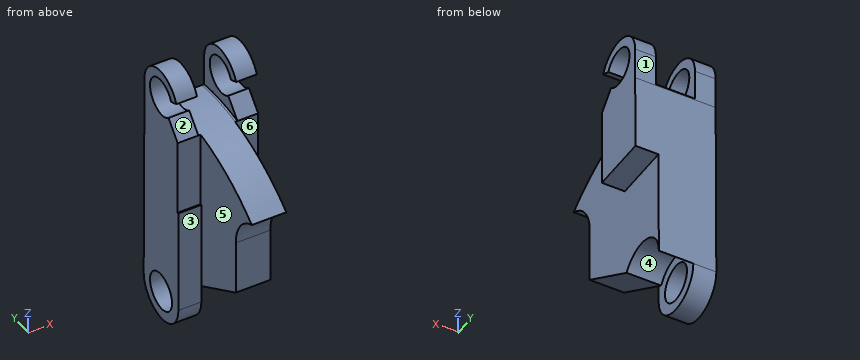
Autodesk Inventor part; units mm, degrees
ref_plane "YZ Plane" through (0, 0, 0) normal (1, 0, 0) x (0, 1, 0)
ref_plane "XZ Plane" through (0, 0, 0) normal (0, 1, 0) x (-1, 0, 0)
ref_plane "XY Plane" through (0, 0, 0) normal (0, 0, 1) x (1, 0, 0)
sketch "スケッチ1" plane through (0, 0, 0) normal (1, 0, 0) x (0, 1, 0)
  line L0 (0, 0) -> (0, 6)
  line L1 (0, 6) -> (0, -6)
  line L2 (0, 0) -> (11.5, 0)
  line L3 (11.5, 0) -> (11.5, 9.5)
  line L4 (11.5, 9.5) -> (11.5, -9.5)
  circle A0 centre (0, 6) radius 1.25
  circle A1 centre (0, -6) radius 1.25
  circle A2 centre (11.5, 9.5) radius 1.65
  circle A3 centre (11.5, -9.5) radius 1.65
  circle A4 centre (11.5, 9.5) radius 2.5
  circle A5 centre (11.5, -9.5) radius 2.5
  circle A6 centre (0, 0) radius 2.65
  line L5 (0, 0) -> (-14.6, 0)
  circle A7 centre (-14.6, 0) radius 1.65
  circle A8 centre (-14.6, 0) radius 2.5
  circle A9 centre (0, 6) radius 2
  circle A10 centre (0, -6) radius 2
  line L6 (0, 8) -> (10.6499, 11.851)
  line L7 (0, -8) -> (10.6499, -11.851)
  line L8 (-14.6, 0) -> (-14.6, -2.5)
  line L9 (-14.6, 0) -> (-12.1, 0) construction
  line L10 (-14.6, -2.5) -> (-14.6, 2.5)
  line L11 (-14.6, -2.5) -> (-0.7212, -7.8655)
  line L12 (-14.6, 2.5) -> (-0.7212, 7.8655)
  circle A11 centre (11.5, -9.5) radius 14.9164
  line L13 (11.5, -9.5) -> (0, 0)
  line L14 (11.5, -9.5) -> (0, -2.65)
  line L15 (14, 9.5) -> (14, 6.6979)
  circle A12 centre (11.5, -9.5) radius 16.7294
  circle A13 centre (11.5, -9.5) radius 2.6
  circle A14 centre (11.5, -9.5) radius 16.5
  line L16 (14, 6.6979) -> (14.1, -9.4839)
  line L17 (8.9, -9.5) -> (8.9, 0)
  line L18 (9, 9.5) -> (9, 0)
  line L19 (14.0414, 0) -> (11.5, 0)
  line L20 (0, 2.65) -> (2.65, 2.65)
  line L21 (2.65, 2.65) -> (2.65, 0)
  line L22 (2.65, 2.65) -> (2.65, 4.4258)
  circle A15 centre (0, 0) radius 3.575
  line L23 (0, 3.575) -> (14.0193, 3.575)
  line L24 (0, 3.575) -> (14.0193, 3.575) construction
  circle A16 centre (0, 0) radius 3.7299
  circle A17 centre (11.5, -9.5) radius 11.1866
  line L25 (0, -3.7299) -> (1.8129, -3.7299)
  line L26 (3.7299, 0) -> (3.7299, -4.8717)
  line L27 (3.7299, -3.7299) -> (1.8129, -3.7299)
  circle A18 centre (11.473, -9.4839) radius 9.6471
  line L28 (11.5, 9.5) -> (9.2001, 10.48)
  line L29 (11.5, 9.5) -> (9, 6.8095)
  point P0 (9.3522, -8.2206)
  point P1 (0, 2.65)
  point P2 (12.4812, 7.2006)
  point P3 (14, 6.8095)
  point P4 (0.3158, 2.6311)
  point P5 (9.2662, -8.1695)
  point P6 (1.3228, 3.4875)
  point P7 (2.6248, 2.65)
  point P8 (2.65, 2.6248)
  point P9 (1.3732, -3.4679)
  point P10 (3.1849, -4.5471)
  point P11 (11.5, 7.2294)
  point P12 (9, 7.0415)
  point P13 (9.9821, 10.1468)
  point P14 (11.5, 7.85)
  point P15 (9.2488, 7.0772)
  point P16 (10.3768, 8.2913)
  dimension "d9" = 5
  dimension "d32" = 7.15
  dimension "d0" = 6
  dimension "d1" = 12
  dimension "d2" = 11.5
  dimension "d3" = 9.5
  dimension "d4" = 19
  dimension "d5" = 2.5
  dimension "d6" = 3.3
  dimension "d7" = 3.3
  dimension "d8" = 5
  dimension "d10" = 5.3
  dimension "d11" = 14.6
  dimension "d12" = 3.3
  dimension "d13" = 5
  dimension "d14" = 4
  dimension "d15" = 4
  dimension "d16" = 90
  dimension "d21" = 5.2
  dimension "d22" = 33
  dimension "d33" = 0
extrude "押し出し3" add sketch "スケッチ1" along normal blind 3 contours L23 L22 L20 A16 A14 | A14 L22 L23 | L18 A11 L23 L22 A14 | A14 L3 A11 L18 | L23 A11 A16 L21 L22 | A14 L15 L16 A11 L3 | L18 L23 A11 | A11 L3 L23 L18 | L23 L18 A17 L2 A16 A11 | L2 A17 L26 | A11 L16 L23 L3 | L23 L3 A17 L18 | A17 L18 L2 | L2 L17 A18 L13 L26 A17 | L13 A18 L26 | L23 L16 A17 L3 | A17 L3 A18 L2 L18 | L2 A18 L17 | A18 L17 L13 | L13 L17 L14 L26 A18 | A17 L16 L19 A18 L3 | A18 L2 L4 A13 L13 L17 | L13 A13 L14 L17 | A18 L19 L3 | L3 L2 A18 | L19 A18 L16 A13 L4 | L19 L16 A18
extrude "押し出し4" add sketch "スケッチ1" against normal blind 2 contours L29 A4 A12 | A12 A4 A14 L29 | A14 L3 A11 L18 | A12 L3 A4 | A4 L29 A2 L3 A12 | A4 A12 L3 A2 L28 | A14 L15 L16 A11 L3 | L3 A12 A4 | A4 A12 L15 A14 | A11 L3 L23 L18 | A11 L16 L23 L3 | A4 L15 A12 | L23 L3 A17 L18 | L23 L16 A17 L3 | A17 L3 A18 L2 L18 | L2 A18 L17 | A17 L16 L19 A18 L3 | A18 L2 L4 A13 L13 L17 | L13 A13 L14 L17 | A18 L19 L3 | L3 L2 A18 | A13 L4 A5 L13 | L13 A5 L14 A13 | L14 A13 L17 | L19 A18 L16 A13 L4 | L19 L16 A18 | A13 L14 A5 L7 | L7 A5 L4 A13 | L13 A3 L14 A5 | A5 L4 A3 L13 | A5 L14 A3 L4
sketch "スケッチ3" plane through (3, 0, 0) normal (1, 0, 0) x (0, 0, -1)
  line L0 (0, 0) -> (0, 11.5)
  line L1 (0, 11.5) -> (-9.5, 11.5)
  circle A0 centre (-9.5, 11.5) radius 1.65
  circle A1 centre (-9.5, 11.5) radius 2.5
  line L2 (-10.1468, 9.9821) -> (-10.48, 9.2001)
  line L3 (-9.5, 11.5) -> (-10.48, 9.2001)
  line L4 (-9.5, 11.5) -> (-6.8095, 9)
  arc A2 (-6.8095, 14) -> (-3.4875, 1.3228) centre (9.5, 11.5) ccw
  line L5 (0, 9) -> (-6.8095, 9)
  line L6 (-6.8095, 9) -> (0, 9)
  line L7 (0, 9) -> (0, 14.0414)
  line L8 (9.4839, 14.1) -> (-6.6979, 14)
  line L9 (-9.5, 14) -> (-6.6979, 14)
  line L10 (-9.5, 14) -> (0, 14.0414)
  point P0 (-8.2913, 10.3768)
  dimension "d37" = 3.3
  dimension "d34" = 11.5
  dimension "d35" = 9.5
  dimension "d36" = 90
  dimension "d38" = 5
extrude "押し出し6" add sketch "スケッチ3" along normal blind 2 contours L5 A2 L1 L0 | L1 A2 L9 L8 L7 | L4 A1 A2 | A1 L4 A0 L1 | L1 A0 L2 A1 | A1 L9 A2
extrude "押し出し7" cut sketch "スケッチ1" against normal blind 0.2 contours L29 A4 A12 | A12 A4 A14 L29 | A12 L3 A4 | A4 L29 A2 L3 A12 | A4 A12 L3 A2 L28 | L3 A12 A4 | A4 A12 L15 A14 | A4 L15 A12
extrude "押し出し8" cut sketch "スケッチ3" along normal blind 0.2 contours L4 A1 A2 | A1 L4 A0 L1 | L1 A0 L2 A1 | A1 L9 A2
properties part number "ikafly2c7"
Source: CAD feature listing. Evaluate the final solid. Frame: model axes, mm. Face numbers are marked on the shaded views. A direction names the side the tool comes from. Round coordinates to 2 decimals unless told otherwise and drop trailing zeros. Loops run counter-clockwise (first coordinate to the right, second up) from the corner with the lowest first, then second, coordinate; pieces in that order, holes last. Notation, with made-up numbers: (-24.5, 54) -> (15.5, 54) arc R34 ccw to (15.5, 85) -> close; hole circle Ø2 at (52.5, 77). An arc over 180 degrees is marked (long way). Answer as a JSON object with one key per item and string values. Group by question number.
Q1. Mould query, pull axis Y, two halves, no side actions, for the marked faces 4, 5 and 6. Classes: pulls with the +Y half, pulls with the -Y half, needs draft (parallel to the pull), parting line crosses it, or undercut.
Q2. Section query B-B (z = -9.75). Output: boundary loops of the cut face in (x, y).
Q3. Section query D-D (x = 4.25). Output: boundary loops of the cut face in (y, z).
Q4. Contact query for flat-ended pins moving along their axis: P1, Ø1.5, axis at x = 1.5, z = -1.5, coming from the -Y side; P2, Ø3, axis at x = 1, z = 8.5, coming from the +Y side; P3, Ø2, axis at x = -1.5, z = 3, coming from the -Y side; P4, Ø2.5, axis at y = 11.5, z = 9.5, coming from the -X side. Output: stop coordinate, or through.
Q5. Access query for the marked faces 1, 2 and 3. Directions: +Z, -Z, +X, -X, +Y, -Y. A direction counts if a zero-diameter tool reaches every point of the face in a straight line with its end or side. Return the directions, or none.
Q6. Section query A-A (y = 11.5). Output: boundary loops of the cut face in (x, z), plus the area to 3 significant figures.
Q7. Section query C-C (y = 9.5). Output: boundary loops of the cut face in (x, z), plus the area to 3 significant figures.
Q8. Ray query, line 1 (Z direction, x = -0.75, y = 11.5); line 2 (Z direction, x = 4.15, y = 11.5); line 3 (Y direction, x = -1, z = -9.5). Return the intervals inside material, ascending. Write a range as from..to.
Completed:
{
 "1": {"face 4": "undercut", "face 5": "needs draft", "face 6": "pulls with the -Y half"},
 "2": {"outline": "(-2, 8.91) -> (0, 8.91) -> (0, 9.87) -> (-2, 9.87) -> close; (-2, 13.13) -> (0, 13.13) -> (0, 14.09) -> (-2, 14.09) -> close"},
 "3": {"outline": "(9, 0) -> (14.04, 0) -> (14, 6.7) -> (14, 9.5) arc R2.5 ccw to (9.2, 10.48) -> (9.98, 10.15) arc R1.65 cw (long way) to (10.38, 8.29) -> (9, 6.81) -> close"},
 "4": {"P1": "y = 3.73", "P2": "y = 14", "P3": "y = 9", "P4": "through"},
 "5": {"face 1": "+Z, +X, -X, +Y", "face 2": "+X, -X, -Y", "face 3": "+Z, -Z, -X, -Y"},
 "6": {"outline": "(-2, -12.1) -> (0, -12.1) -> (0, -11.15) -> (-2, -11.15) -> close; (-2, -7.85) -> (0, -7.85) -> (0, -6.9) -> (3, -6.9) -> (3, 0) -> (5, 0) -> (5, 7.85) -> (3.2, 7.85) -> (3.2, 7) -> (-0.2, 7) -> (-0.2, 7.85) -> (-2, 7.85) -> close; (-2, 11.15) -> (-0.2, 11.15) -> (-0.2, 12) -> (-2, 12) -> close; (3.2, 11.15) -> (5, 11.15) -> (5, 12) -> (3.2, 12) -> close", "area": "93.4 mm²"},
 "7": {"outline": "(-2, -11.16) -> (0, -11.16) -> (0, -7.84) -> (3, -7.84) -> (3, 0) -> (5, 0) -> (5, 7.35) -> (3.2, 7.35) -> (3.2, 6.88) -> (-0.2, 6.88) -> (-0.2, 7.35) -> (-2, 7.35) -> close; (-2, 10.35) -> (-0.2, 10.35) -> (-0.2, 11) -> (-2, 11) -> close; (3.2, 10.35) -> (5, 10.35) -> (5, 11) -> (3.2, 11) -> close", "area": "98.0 mm²"},
 "8": {"line 1": "-12.1..-11.15, -7.85..7.85, 11.15..12", "line 2": "0..7.85, 11.15..12", "line 3": "8.9..9.85, 13.15..14.1"}
}
